```python
from build123d import *

# Parameters (mm, degrees)
ESBO_O1_W             = 70
ESBO_O1_H             = 50
EXTRUS_O1_DEPTH       = 60
CORTE_EXTRUS_O2_DEPTH = 35


with BuildPart() as part:
    # Esboço1 → Extrusão1 (new body)
    with BuildSketch(Plane(origin=(0, 0, 0), x_dir=(1, 0, 0), z_dir=(0, 1, 0))):
        Rectangle(ESBO_O1_W, ESBO_O1_H)
    extrude(amount=EXTRUS_O1_DEPTH)

    # Esboço5 → Corte-extrusão2 (cut)
    with BuildSketch(Plane.ZY.offset(35)):
        Polygon((0, 60), (25, 30), (25, 60), align=None)
    extrude(amount=-CORTE_EXTRUS_O2_DEPTH, mode=Mode.SUBTRACT)

    # Corte de superfície4
    split(bisect_by=Plane(origin=(24.299305734, 28.349190023, 34.019028028), x_dir=(-0.876685828, 0.30796926, 0.369563112), z_dir=(-0.481063363, -0.56124059, -0.673488708)), keep=Keep.TOP)


solid = part.part
```
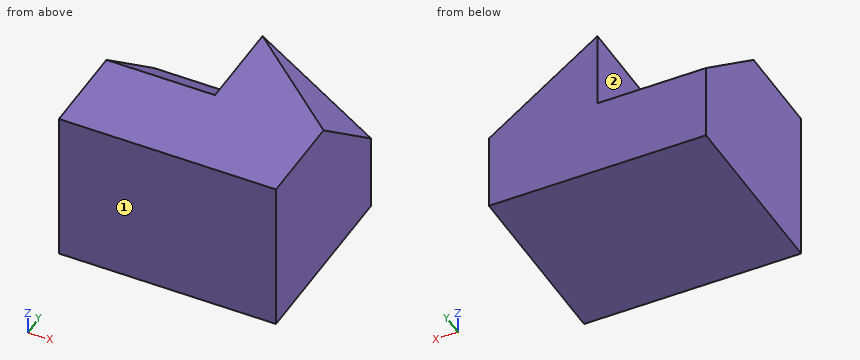
Can you work these out from the model? Positions are in its coordinate system, mm. Face numbers are marked on the shaded views. A direction names the side the tool comes from. Coordinates: 2 decimals unless noted, no trailing zeros. Loops run counter-clockwise (first coordinate to the right, second up) from the corner with the lowest first, then second, coordinate; pieces in that order, holes last. Notation, with made-up numbers: (42, 14) - (89, 14) arc R25 cw to (89, 47) - close; hole circle Ø2 at (48, 34.5). An arc over 180 degrees is marked (long way). Answer as CSV lines item,"result". Start each with the question number.
1) Suppose I cut it at B-B (y = 36). Please give me the cut outline in (x, z).
2) Which directions (+Z, -Z, +X, -X, +Y, -Y) give clear straight access to the entire face, cutting with the end or side of a thin tool? Please do the marked faces 1 and 2.
3) Suppose I cut it at A-A (z = 20.5). Please give me the cut outline in (x, y).
4) Suppose I cut it at D-D (x = -1.5). Please give me the cut outline in (y, z).
5) I need wall thicknesses on line 1 (Z direction, x = -1, y = 39); line 2 (Z direction, x = -14, y = 39.5); line 3 (Y direction, x = -4, z = 16.5). Which ranges of each line are inside material? Lowest first, please. Write a range as from..to.
6) Suppose I cut it at C-C (x = 17.5). Please give me the cut outline in (y, z).
7) For pin 1 (6 mm diameter, centred on x = -26.5, z = 17, fed in from +Y); pin 2 (1 mm diameter, centred on x = -21, y = 40.5, fed in from +Z); pin 3 (1 mm diameter, centred on y = 41.5, z = 17.5, fed in from +X), each with a flat end and sliding along its axis, tell me the tip position at first contact or that it passes through.
Check result:
1,outline,"(-35, -25) - (35, -25) - (35, 20) - (28, 25) - (0, 25) - (0, 20) - (-35, 20) - close"
2,face 1,"+Z, -Z, +X, -X, -Y"
2,face 2,"+Z, -X, +Y"
3,outline,"(-35, 0) - (35, 0) - (35, 35.4) - (6.3, 60) - (0, 60) - (0, 35.4) - (-35, 35.4) - close"
4,outline,"(0, -25) - (60, -25) - (60, 0) - (30, 25) - (0, 25) - close"
5,line 1,"z = -25..17.5"
5,line 2,"z = -25..17.08"
5,line 3,"y = 0..40.2"
6,outline,"(0, -25) - (60, -25) - (60, 12.5) - (45, 25) - (0, 25) - close"
7,pin 1,"stops at y = 43.2"
7,pin 2,"stops at z = 16.67"
7,pin 3,"stops at x = 32.99"
